```python
from build123d import *

# Parameters (mm, degrees)
SKETCH1_R           = 2.8575
BOSS_EXTRUDE1_DEPTH = 3.5052
CUT_EXTRUDE1_DEPTH  = 1.9558
SKETCH3_R           = 1.7145
BOSS_EXTRUDE2_DEPTH = 34.925


with BuildPart() as part:
    # Sketch1 → Boss-Extrude1 (new body)
    with BuildSketch(Plane(origin=(0, 0, 0), x_dir=(1, 0, 0), z_dir=(0, 1, 0))):
        Circle(SKETCH1_R)
    extrude(amount=BOSS_EXTRUDE1_DEPTH)

    # Sketch2 → Cut-Extrude1 (cut)
    with BuildSketch(Plane.XZ):
        Polygon((1.603951217, 0), (0.801975608, 1.3890625), (-0.801975608, 1.3890625), (-1.603951217, 0), (-0.801975608, -1.3890625), (0.801975608, -1.3890625), align=None)
    extrude(amount=-CUT_EXTRUDE1_DEPTH, mode=Mode.SUBTRACT)

    # Sketch3 → Boss-Extrude2 (add)
    with BuildSketch(Plane(origin=(0, 3.5052, 0), x_dir=(1, 0, 0), z_dir=(0, 1, 0))):
        Circle(SKETCH3_R)
    extrude(amount=BOSS_EXTRUDE2_DEPTH)


solid = part.part
```
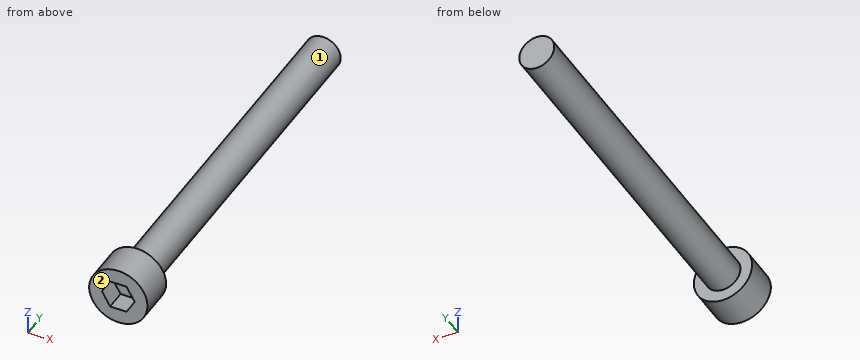
Check sheet for the modelled part. Datum: model origin and axes. Units: mm. Face numbers are marked on the shaded views. A direction names the side the tool comes from. Coordinates: 2 decimals unless noted, no trailing zeros. Order: outer loops, then holes, each group sorted by start corner. A loop starts at its lowest first (then second) coordinate and runs counter-clockwise, first axis right, second up. Notation, with made-up numbers: M -14.5,71 L 2.5,71 A33 cw 2.5,101 Z; hole C 35,59 d6. An arc over 180 degrees is marked long. Write each question's results on one line, items separated by ' | '. Start each with the question number.
1. Access from +Z, -Z, +X, -X, +Y, -Y to the whole of each face (thin tool, end or side, straight path). Record for the marked faces 1 and 2.
2. Cross-section at D-D on y = 11. Record the cut outline in (x, z), and give its area (3 significant figures).
3. Cross-section at A-A on x = 0. Record the cut outline in (y, z).
4. Material ranges on probe 1 along Y at (x, z) = (-0.05, 1.8); probe 2 along Y at (x, z) = (-0.1, 1.3); probe 3 along Z at (x, y) = (-1, 31), recorded low to high.
5. Cross-section at C-C on z = -2.45. Record the cut outline in (x, y), and give its area (3 significant figures).
6. Go/stop test with flat-tipped pins: P1, Ø3, axis at y = 24, z = -2, coming from the -X side; P2, Ø0.8, axis at x = 0.5, z = 0, coming from the -Y side; P3, Ø1.5, axis at y = 18, z = -0.5, coming from the -X side. Record where each tip stops, or that it passes through.
7. Cross-section at B-B on y = 3. Record the cut outline in (x, z) (1 decimal).
Checks:
1) face 1: +Y | face 2: +Z, -Z, +X, -X, -Y
2) outline: C 0,0 d3.43 | area: 9.23 mm²
3) outline: M 0,-2.86 L 3.51,-2.86 L 3.51,-1.71 L 38.43,-1.71 L 38.43,1.71 L 3.51,1.71 L 3.51,2.86 L 0,2.86 L 0,1.39 L 1.96,1.39 L 1.96,-1.39 L 0,-1.39 Z
4) probe 1: y = 0 to 3.51 | probe 2: y = 1.96 to 38.43 | probe 3: z = -1.39 to 1.39
5) outline: M -1.47,0 L 1.47,0 L 1.47,3.51 L -1.47,3.51 Z | area: 10.3 mm²
6) P1: stops at x = -1.64 | P2: stops at y = 1.96 | P3: stops at x = -1.71
7) outline: C 0,0 d5.7
